Geometry check sheet. Reference: the model listing, model coordinates, mm. A direction names the side the tool comes from. Coordinates: 2 decimals unless noted, no trailing zeros. Write each loop counter-clockwise with the first axis right and the second up, starting at its lowest first coordinate (ties: lowest second). Pieces come first, ordered by that corner, then holes. Notation, with made-up numbers: M -4,18 L 12,18 A31 cw 12,48 Z; hole C 48.25,14 d3. An arc over 180 degrees is marked long. Write item = value, one per line. Start each with the question number.
```python
from build123d import *

# Parameters (mm, degrees)
SKETCH1_W             = 25
SKETCH1_H             = 450
BOSS_EXTRUDE2_DEPTH   = 25
BOSS_EXTRUDE2_2_DEPTH = 25
SKETCH2_W             = 25
SKETCH2_H             = 25
BOSS_EXTRUDE3_DEPTH   = 200
SKETCH3_W             = 25
SKETCH3_H             = 450
BOSS_EXTRUDE4_DEPTH   = 25
SKETCH5_W             = 25
SKETCH5_H             = 25
BOSS_EXTRUDE5_DEPTH   = 200
SKETCH6_W             = 25
SKETCH6_H             = 450
BOSS_EXTRUDE6_DEPTH   = 25
SKETCH7_W             = 800
SKETCH7_H             = 25
BOSS_EXTRUDE7_DEPTH   = 25
SKETCH8_W             = 350
SKETCH8_H             = 25
BOSS_EXTRUDE8_DEPTH   = 25
SKETCH9_W             = 25
SKETCH9_H             = 425
BOSS_EXTRUDE9_DEPTH   = 25
SKETCH10_W            = 25
SKETCH10_H            = 25
BOSS_EXTRUDE10_DEPTH  = 800
BOSS_EXTRUDE13_REACH  = 532.919
SKETCH14_W            = 25
SKETCH14_H            = 25
SKETCH15_W            = 185
SKETCH15_H            = 450
BOSS_EXTRUDE14_DEPTH  = 6
BOSS_EXTRUDE15_DEPTH  = 6
CUT_EXTRUDE2_REACH    = 511.717
SKETCH19_R            = 4
CUT_EXTRUDE4_REACH    = 530.404
SKETCH20_R            = 4
SKETCH21_R            = 5
SKETCH21_R_2          = 2.5
CUT_EXTRUDE5_DEPTH    = 10
BOSS_EXTRUDE16_REACH  = 652.961
SKETCH24_W            = 25
SKETCH24_H            = 25
SKETCH25_R            = 2.5
CUT_EXTRUDE6_DEPTH    = 10


with BuildPart() as part:
    # Sketch1 → Boss-Extrude2 (new body)
    with BuildSketch(Plane(origin=(0, 0, 0), x_dir=(1, 0, 0), z_dir=(0, 1, 0))):
        with Locations((-412.5, 0)):
            Rectangle(SKETCH1_W, SKETCH1_H)
    extrude(amount=BOSS_EXTRUDE2_DEPTH)

    # Sketch2 → Boss-Extrude3 (add)
    with BuildSketch(Plane(origin=(0, 25, 0), x_dir=(1, 0, 0), z_dir=(0, 1, 0))):
        with Locations((-412.5, 212.5)):
            Rectangle(SKETCH2_W, SKETCH2_H)
        with Locations((-412.5, -212.5)):
            Rectangle(SKETCH2_W, SKETCH2_H)
    extrude(amount=BOSS_EXTRUDE3_DEPTH)

    # Sketch3 → Boss-Extrude4 (add)
    with BuildSketch(Plane(origin=(0, 225, 0), x_dir=(1, 0, 0), z_dir=(0, 1, 0))):
        with Locations((-412.5, 0)):
            Rectangle(SKETCH3_W, SKETCH3_H)
    extrude(amount=BOSS_EXTRUDE4_DEPTH)



with BuildPart() as body_2:
    # Sketch1 → Boss-Extrude2 2 (new body)
    with BuildSketch(Plane(origin=(0, 0, 0), x_dir=(1, 0, 0), z_dir=(0, 1, 0))):
        with Locations((412.5, 0)):
            Rectangle(SKETCH1_W, SKETCH1_H)
    extrude(amount=BOSS_EXTRUDE2_2_DEPTH)

    # Sketch5 → Boss-Extrude5 (add)
    with BuildSketch(Plane(origin=(0, 25, 0), x_dir=(1, 0, 0), z_dir=(0, 1, 0))):
        with Locations((412.5, 212.5)):
            Rectangle(SKETCH5_W, SKETCH5_H)
        with Locations((412.5, -212.5)):
            Rectangle(SKETCH5_W, SKETCH5_H)
    extrude(amount=BOSS_EXTRUDE5_DEPTH)

    # Sketch6 → Boss-Extrude6 (add)
    with BuildSketch(Plane(origin=(0, 225, 0), x_dir=(1, 0, 0), z_dir=(0, 1, 0))):
        with Locations((412.5, 0)):
            Rectangle(SKETCH6_W, SKETCH6_H)
    extrude(amount=BOSS_EXTRUDE6_DEPTH)


with BuildPart() as part_1:
    add(part.part)

    add(body_2.part)  # Boss-Extrude7 merges body 2
    # Sketch7 → Boss-Extrude7 (add)
    with BuildSketch(Plane(origin=(0, 250, 0), x_dir=(1, 0, 0), z_dir=(0, 1, 0))):
        with Locations((0, 212.5)):
            Rectangle(SKETCH7_W, SKETCH7_H)
        with Locations((0, -212.5)):
            Rectangle(SKETCH7_W, SKETCH7_H)
    extrude(amount=-BOSS_EXTRUDE7_DEPTH)

    # Sketch8 → Boss-Extrude8 (add)
    with BuildSketch(Plane(origin=(0, 0, 0), x_dir=(-1, 0, 0), z_dir=(0, -1, 0))):
        with Locations((-225, 212.5)):
            Rectangle(SKETCH8_W, SKETCH8_H)
        with Locations((-225, -212.5)):
            Rectangle(SKETCH8_W, SKETCH8_H)
    extrude(amount=-BOSS_EXTRUDE8_DEPTH)

    # Sketch9 → Boss-Extrude9 (add)
    with BuildSketch(Plane(origin=(0, 0, 0), x_dir=(-1, 0, 0), z_dir=(0, -1, 0))):
        with Locations((-62.5, -12.5)):
            Rectangle(SKETCH9_W, SKETCH9_H)
    extrude(amount=-BOSS_EXTRUDE9_DEPTH)

    # Sketch10 → Boss-Extrude10 (add)
    with BuildSketch(Plane.ZY.offset(-400)):
        with Locations((212.5, 187.5)):
            Rectangle(SKETCH10_W, SKETCH10_H)
        with Locations((-212.5, 187.5)):
            Rectangle(SKETCH10_W, SKETCH10_H)
    extrude(amount=BOSS_EXTRUDE10_DEPTH)

    # Sketch14 → Boss-Extrude13 (add, up to next)
    with BuildSketch(Plane(origin=(0, 25, 0), x_dir=(1, 0, 0), z_dir=(0, 1, 0)), mode=Mode.PRIVATE) as boss_extrude13_sk1:
        with Locations((62.5, 212.5)):
            Rectangle(SKETCH14_W, SKETCH14_H)
    boss_extrude13_tool1 = extrude(boss_extrude13_sk1.sketch, amount=BOSS_EXTRUDE13_REACH, mode=Mode.PRIVATE) - part_1.part
    # Sketch14 → Boss-Extrude13 (add, up to next)
    with BuildSketch(Plane(origin=(0, 25, 0), x_dir=(1, 0, 0), z_dir=(0, 1, 0)), mode=Mode.PRIVATE) as boss_extrude13_sk2:
        with Locations((62.5, -212.5)):
            Rectangle(SKETCH14_W, SKETCH14_H)
    boss_extrude13_tool2 = extrude(boss_extrude13_sk2.sketch, amount=BOSS_EXTRUDE13_REACH, mode=Mode.PRIVATE) - part_1.part
    add(boss_extrude13_tool1.solids().sort_by_distance((62.5, 25, -212.5))[0])
    add(boss_extrude13_tool2.solids().sort_by_distance((62.5, 25, 212.5))[0])

    # Sketch15 → Boss-Extrude14 (add)
    with BuildSketch(Plane.XZ.offset(-175)):
        with Locations((-175, 0)):
            Rectangle(SKETCH15_W, SKETCH15_H)
    extrude(amount=BOSS_EXTRUDE14_DEPTH)

    # Sketch18 → Boss-Extrude15 (add)
    with BuildSketch(Plane(origin=(0, 25, 0), x_dir=(1, 0, 0), z_dir=(0, 1, 0))):
        Polygon((194.602808883, 225), (313.254235522, 225), (344.602808883, 193.65142664), (344.602808883, -193.65142664), (313.254235522, -225), (194.602808883, -225), align=None)
    extrude(amount=BOSS_EXTRUDE15_DEPTH)

    # Sketch19 → Cut-Extrude2 (cut, up to next)
    with BuildSketch(Plane.XZ.offset(-169), mode=Mode.PRIVATE) as cut_extrude2_sk1:
        with Locations(Location((-227.5, 212.5, 0), (0, 0, 270))):
            Circle(SKETCH19_R)
    cut_extrude2_tool1 = extrude(cut_extrude2_sk1.sketch, amount=-CUT_EXTRUDE2_REACH, mode=Mode.PRIVATE) & part_1.part
    # Sketch19 → Cut-Extrude2 (cut, up to next)
    with BuildSketch(Plane.XZ.offset(-169), mode=Mode.PRIVATE) as cut_extrude2_sk2:
        with Locations(Location((-122.5, 212.5, 0), (0, 0, 270))):
            Circle(SKETCH19_R)
    cut_extrude2_tool2 = extrude(cut_extrude2_sk2.sketch, amount=-CUT_EXTRUDE2_REACH, mode=Mode.PRIVATE) & part_1.part
    # Sketch19 → Cut-Extrude2 (cut, up to next)
    with BuildSketch(Plane.XZ.offset(-169), mode=Mode.PRIVATE) as cut_extrude2_sk3:
        with Locations(Location((-227.5, -212.5, 0), (0, 0, 270))):
            Circle(SKETCH19_R)
    cut_extrude2_tool3 = extrude(cut_extrude2_sk3.sketch, amount=-CUT_EXTRUDE2_REACH, mode=Mode.PRIVATE) & part_1.part
    # Sketch19 → Cut-Extrude2 (cut, up to next)
    with BuildSketch(Plane.XZ.offset(-169), mode=Mode.PRIVATE) as cut_extrude2_sk4:
        with Locations(Location((-122.5, -212.5, 0), (0, 0, 270))):
            Circle(SKETCH19_R)
    cut_extrude2_tool4 = extrude(cut_extrude2_sk4.sketch, amount=-CUT_EXTRUDE2_REACH, mode=Mode.PRIVATE) & part_1.part
    add(cut_extrude2_tool1.solids().sort_by_distance((-227.5, 169, 212.5))[0], mode=Mode.SUBTRACT)
    add(cut_extrude2_tool2.solids().sort_by_distance((-122.5, 169, 212.5))[0], mode=Mode.SUBTRACT)
    add(cut_extrude2_tool3.solids().sort_by_distance((-227.5, 169, -212.5))[0], mode=Mode.SUBTRACT)
    add(cut_extrude2_tool4.solids().sort_by_distance((-122.5, 169, -212.5))[0], mode=Mode.SUBTRACT)

    # Sketch20 → Cut-Extrude4 (cut, up to next)
    with BuildSketch(Plane(origin=(0, 31, 0), x_dir=(1, 0, 0), z_dir=(0, 1, 0)), mode=Mode.PRIVATE) as cut_extrude4_sk1:
        with Locations(Location((264.602808883, 212.5, 0), (0, 0, 270))):
            Circle(SKETCH20_R)
    cut_extrude4_tool1 = extrude(cut_extrude4_sk1.sketch, amount=-CUT_EXTRUDE4_REACH, mode=Mode.PRIVATE) & part_1.part
    # Sketch20 → Cut-Extrude4 (cut, up to next)
    with BuildSketch(Plane(origin=(0, 31, 0), x_dir=(1, 0, 0), z_dir=(0, 1, 0)), mode=Mode.PRIVATE) as cut_extrude4_sk2:
        with Locations(Location((264.602808883, -212.5, 0), (0, 0, 90))):
            Circle(SKETCH20_R)
    cut_extrude4_tool2 = extrude(cut_extrude4_sk2.sketch, amount=-CUT_EXTRUDE4_REACH, mode=Mode.PRIVATE) & part_1.part
    add(cut_extrude4_tool1.solids().sort_by_distance((264.602809, 31, -212.5))[0], mode=Mode.SUBTRACT)
    add(cut_extrude4_tool2.solids().sort_by_distance((264.602809, 31, 212.5))[0], mode=Mode.SUBTRACT)

    # Sketch21 → Cut-Extrude5 (cut)
    with BuildSketch(Plane.XZ.offset(-169)):
        with Locations(Location((-175, 0, 0), (0, 0, 270))):
            Circle(SKETCH21_R)
        with Locations(Location((-209.626678733, 34.626678733, 0), (0, 0, 270))):
            Circle(SKETCH21_R_2)
        with Locations(Location((-140.373321267, 34.626678733, 0), (0, 0, 270))):
            Circle(SKETCH21_R_2)
        with Locations(Location((-140.373321267, -34.626678733, 0), (0, 0, 270))):
            Circle(SKETCH21_R_2)
        with Locations(Location((-209.626678733, -34.626678733, 0), (0, 0, 270))):
            Circle(SKETCH21_R_2)
    extrude(amount=-CUT_EXTRUDE5_DEPTH, mode=Mode.SUBTRACT)

    # Sketch24 → Boss-Extrude16 (add, up to next)
    with BuildSketch(Plane.XY.offset(-200), mode=Mode.PRIVATE) as boss_extrude16_sk1:
        with Locations((62.5, 187.5)):
            Rectangle(SKETCH24_W, SKETCH24_H)
    boss_extrude16_tool1 = extrude(boss_extrude16_sk1.sketch, amount=BOSS_EXTRUDE16_REACH, mode=Mode.PRIVATE) - part_1.part
    # Sketch24 → Boss-Extrude16 (add, up to next)
    with BuildSketch(Plane.XY.offset(-200), mode=Mode.PRIVATE) as boss_extrude16_sk2:
        with Locations((62.5, 237.5)):
            Rectangle(SKETCH24_W, SKETCH24_H)
    boss_extrude16_tool2 = extrude(boss_extrude16_sk2.sketch, amount=BOSS_EXTRUDE16_REACH, mode=Mode.PRIVATE) - part_1.part
    add(boss_extrude16_tool1.solids().sort_by_distance((62.5, 187.5, -200))[0])
    add(boss_extrude16_tool2.solids().sort_by_distance((62.5, 237.5, -200))[0])

    # Sketch25 → Cut-Extrude6 (cut)
    with BuildSketch(Plane(origin=(0, 31, 0), x_dir=(1, 0, 0), z_dir=(0, 1, 0))):
        with Locations(Location((241.318537635, 28.284271247, 0), (0, 0, 270))):
            Circle(SKETCH25_R)
        with Locations(Location((297.88708013, 28.284271247, 0), (0, 0, 270))):
            Circle(SKETCH25_R)
        with Locations(Location((297.88708013, -28.284271247, 0), (0, 0, 270))):
            Circle(SKETCH25_R)
        with Locations(Location((241.318537635, -28.284271247, 0), (0, 0, 270))):
            Circle(SKETCH25_R)
    extrude(amount=-CUT_EXTRUDE6_DEPTH, mode=Mode.SUBTRACT)


solid = part_1.part
```
Q1. Cross-section at C-C on y = 51. Enter the section's corners in (x, z).
Q2. Draft check along X on faces 1 (the face through (328.709, 27.958, -209.545)), 2 (the face through (425, 226, 34)), 3 (the face through (412, 25, -3)). Enter one of: pulls with the +X half, pulls with the -X half, needs draft (parallel to the pull), parting line crosses it, or undercut.
Q3. Set-up check for faces 4 (the face through (75, 99, 213)), 5 (the face through (288, 176, 200)), 6 (the face through (-224, 176, 200)), 7 (the face through (-178, 238, -200)): record each of +Z, -Z, +X, -X, +Y, -Y from which the full face is reachable in a straight line by a thin tool's end or side.
Q4. Cross-section at A-A on x = -42. Enter the section's corners in (y, z).
Q5. Cross-section at D-D on x = -252.5. Enter the section's corners in (y, z).
Q6. Gauge pin test, flat ends, axial feed: pin 1 (6 mm diameter, centred on x = 297.89, z = -28.28, fed in from +Y); pin 2 (8 mm diameter, centred on x = -175.5, z = 16, fed in from -Y); pin 3 (5 mm diameter, centred on y = 173.5, z = -29.5, fed in from -X); pin 4 (8 mm diameter, centred on x = 190.5, z = -102, fed in from -Y). Record the tip position at first contact, or that the pin passes through.
Q7. Scan lines: L1, parallel to X at y = 179, z = -212; L2, parallel to X at y = 238.5, z = -91.5; L3, parallel to Z at x = -227, y = 176. Record each from-to range of solid material in increasing order.
Q8. Cross-section at B-B on x = 157. Enter the section's corners in (y, z), and give its area (3 significant figures).
Values found:
q1.outline = M -425,-225 L -400,-225 L -400,-200 L -425,-200 Z; M -425,200 L -400,200 L -400,225 L -425,225 Z; M 50,-225 L 75,-225 L 75,-200 L 50,-200 Z; M 50,200 L 75,200 L 75,225 L 50,225 Z; M 400,-225 L 425,-225 L 425,-200 L 400,-200 Z; M 400,200 L 425,200 L 425,225 L 400,225 Z
q2.face_1 = undercut
q2.face_2 = pulls with the +X half
q2.face_3 = needs draft
q3.face_4 = +Z, -Z
q3.face_5 = +X
q3.face_6 = -X
q3.face_7 = +Y
q4.outline = M 175,-225 L 200,-225 L 200,-200 L 175,-200 Z; M 175,200 L 200,200 L 200,225 L 175,225 Z; M 225,-225 L 250,-225 L 250,-200 L 225,-200 Z; M 225,200 L 250,200 L 250,225 L 225,225 Z
q5.outline = M 169,-225 L 200,-225 L 200,-200 L 175,-200 L 175,200 L 200,200 L 200,225 L 169,225 Z; M 225,-225 L 250,-225 L 250,-200 L 225,-200 Z; M 225,200 L 250,200 L 250,225 L 225,225 Z
q6.pin_1 = 31
q6.pin_2 = 169
q6.pin_3 = -267.5
q6.pin_4 = through
q7.L1 = -425 to -231.47, -223.53 to -126.47, -118.53 to 425
q7.L2 = -425 to -400, 50 to 75, 400 to 425
q7.L3 = -225 to -216.47, -208.53 to -200, 200 to 208.53, 216.47 to 225
q8.outline = M 0,-225 L 25,-225 L 25,-200 L 0,-200 Z; M 0,200 L 25,200 L 25,225 L 0,225 Z; M 175,-225 L 200,-225 L 200,-200 L 175,-200 Z; M 175,200 L 200,200 L 200,225 L 175,225 Z; M 225,-225 L 250,-225 L 250,-200 L 225,-200 Z; M 225,200 L 250,200 L 250,225 L 225,225 Z
q8.area = 3,750 mm²
